The model under review builds one solid part; all positions refer to its coordinate system, in mm. Round coordinates to 2 decimals unless told otherwise and drop trailing zeros. Loops run counter-clockwise (first coordinate to the right, second up) from the corner with the lowest first, then second, coordinate; pieces in that order, holes last. Notation, with made-up numbers: M 57,4.25 L 84,4.25 A28 cw 84,34.25 Z; hole C 8,59.5 d7. An arc over 180 degrees is marked long. Answer as a JSON object with one key per item and string values. Group by question number.
Item 1: Consider section B-B (z = 299.5). Give the boundary of the cut face in (x, y).
Item 2: The part is to be moulded in two halves that separate along Z. For faces 1 (the face through (342.01, 3.13, 345.56)), 2 (the face through (127.8, 3.1, -85.7)), 3 (the face through (339.7, 3.1, 127.8)), 4 (the face through (126.2, 3.1, 339.7)), say which applies: +Z half, -Z half, draft (parallel to the pull), parting line (faces both ways), or undercut.
Item 3: Consider section C-C (y = 2.25). Give the boundary of the cut face in (x, z), and give its area (3 significant figures).
Item 4: Insertion check: P1, Ø1, axis at x = 198.5, y = 2.5, coming from the +Z side; P2, Ø1, axis at x = 206.5, y = 1, coming from the -Z side; P3, Ø1.5, axis at y = 3, z = 84, coming from the -X side. Each pin has a flat end and moves straight along its axis. Give the tip position at first contact, or say it passes through.
Item 5: To check wall thickness, follow line 1 (Z direction, x = 254, y = 5.25); line 2 (Z direction, x = 258, y = 1.5). State the ranges of each line that lie inside material, in increasing order.
Item 6: Consider section A-A (x = 254). Give the boundary of the cut face in (y, z), and give its area (3 significant figures).
Item 7: Consider section D-D (z = 153). Give the boundary of the cut face in (x, y), and give its area (3 significant figures).
```python
from build123d import *

# Parameters (mm, degrees)
SKETCH1_R           = 95.25
BOSS_EXTRUDE1_DEPTH = 6.35


with BuildPart() as part:
    # Sketch1 → Boss-Extrude1 (new body)
    with BuildSketch(Plane(origin=(0, 0, 0), x_dir=(1, 0, 0), z_dir=(0, 1, 0))):
        with BuildLine():
            ThreePointArc((74.705882353, 102.703608222), (-89.802561211, 89.802561211), (-102.703608222, -74.705882353))
            ThreePointArc((-102.703608222, -74.705882353), (-85.696133978, -127), (-102.703608222, -179.294117647))
            ThreePointArc((-102.703608222, -179.294117647), (-89.802561211, -343.802561211), (74.705882353, -356.703608222))
            ThreePointArc((74.705882353, -356.703608222), (127, -339.696133978), (179.294117647, -356.703608222))
            ThreePointArc((179.294117647, -356.703608222), (343.802561211, -343.802561211), (356.703608222, -179.294117647))
            ThreePointArc((356.703608222, -179.294117647), (339.696133978, -127), (356.703608222, -74.705882353))
            ThreePointArc((356.703608222, -74.705882353), (343.802561211, 89.802561211), (179.294117647, 102.703608222))
            ThreePointArc((179.294117647, 102.703608222), (127, 85.696133978), (74.705882353, 102.703608222))
        make_face()
        Circle(SKETCH1_R, mode=Mode.SUBTRACT)
        with Locations((254, 0)):
            Circle(SKETCH1_R, mode=Mode.SUBTRACT)
        with Locations((254, -254)):
            Circle(SKETCH1_R, mode=Mode.SUBTRACT)
        with Locations((0, -254)):
            Circle(SKETCH1_R, mode=Mode.SUBTRACT)
    extrude(amount=BOSS_EXTRUDE1_DEPTH)


solid = part.part
```
Geometry results:
{
 "1": {"outline": "M -118.57,0 L -83.68,0 L -83.68,6.35 L -118.57,6.35 Z; M 83.68,0 L 170.32,0 L 170.32,6.35 L 83.68,6.35 Z; M 337.68,0 L 372.57,0 L 372.57,6.35 L 337.68,6.35 Z"},
 "2": {"face 1": "undercut", "face 2": "-Z half", "face 3": "undercut", "face 4": "+Z half"},
 "3": {"outline": "M -102.7,74.71 A127 ccw 74.71,-102.7 A88.9 cw 179.29,-102.7 A127 ccw 356.7,74.71 A88.9 cw 356.7,179.29 A127 ccw 179.29,356.7 A88.9 cw 74.71,356.7 A127 ccw -102.7,179.29 A88.9 cw Z; hole C 0,0 d190.5; hole C 0,254 d190.5; hole C 254,0 d190.5; hole C 254,254 d190.5", "area": "111,000 mm^2"},
 "4": {"P1": "stops at z = 368.47", "P2": "stops at z = -117.98", "P3": "stops at x = -97.21"},
 "5": {"line 1": "z = -127 to -95.25, 95.25 to 158.75, 349.25 to 381", "line 2": "z = -126.94 to -95.17, 95.17 to 158.83, 349.17 to 380.94"},
 "6": {"outline": "M 0,-127 L 6.35,-127 L 6.35,-95.25 L 0,-95.25 Z; M 0,95.25 L 6.35,95.25 L 6.35,158.75 L 0,158.75 Z; M 0,349.25 L 6.35,349.25 L 6.35,381 L 0,381 Z", "area": "806 mm^2"},
 "7": {"outline": "M -89.58,0 L 343.58,0 L 343.58,6.35 L -89.58,6.35 Z", "area": "2,750 mm^2"}
}
